Source: CAD feature listing. Evaluate the final solid. Frame: model axes, mm. Face numbers are marked on the shaded views. A direction names the side the tool comes from. Give positions to 0.01 mm unless a question says otherwise; leave off trailing zeros. Loops run counter-clockwise (first coordinate to the right, second up) from the corner with the lowest first, then second, coordinate; pieces in that order, holes last. Notation, with made-up numbers: (-21.5, 23) - (11.5, 23) arc R11 cw to (11.5, 28) - close; hole circle Ø5 at (9, 44). An arc over 180 degrees is marked (long way). Write each question's results on one line, items separated by ' | '. Start each with the question number.
(1) Cut plane A-A on x = 0. Return the cut outline in (y, z) (3 decimals).
(2) Cut plane B-B on z = -11. Return the cut outline in (x, y), then the cut area to 3 significant figures.
(3) Cut plane D-D on z = -1.5. Return the cut outline in (x, y).
(4) Contact query for flat-ended pins moving along their axis: pin 1 (1 mm diameter, centred on x = 25.5, y = -17, fed in from -Z); pin 2 (6 mm diameter, centred on x = 34.5, z = 1.5, fed in from -Y); pin 3 (4 mm diameter, centred on x = 25, y = -11, fed in from +Z). Output: stop coordinate, or through.
(5) Reachability of the marked faces 1 and 2 from +Z, -Z, +X, -X, +Y, -Y: full face, straight path, thin tool, end or side. Return the list, or none.
(6) Pull-direction query (Z, two-part tool) for the marked faces 3, 4, 5 and 6; classes: pulls with the +Z half, pulls with the -Z half, needs draft (parallel to the pull), parting line crosses it, or undercut.
(7) Material intervals for line 1 along Z through (x, y) = (0, -12) (3 decimals); line 2 along X through (y, z) = (-11, -7); line 3 along X through (y, z) = (-8.5, -1.5), sorted ascending. Write a range as [from, to].
(8) Cut plane C-C on y = -42.5. Return the cut outline in (x, z) (3 decimals), then the cut area to 3 significant figures.
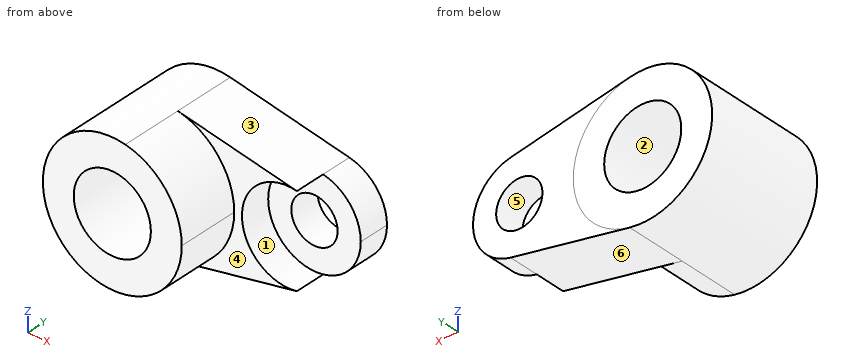
from build123d import *

# Parameters (mm, degrees)
F1_DEPTH = 25.4
F0_R     = 15.875
F2_DEPTH = 50.8
F0_R_2   = 9.525
F3_DEPTH = 12.7


with BuildPart() as f1:
    # F0 (on Front) → F1 (new body)
    with BuildSketch(Plane.XZ):
        with BuildLine():
            ThreePointArc((5.357812, 28.068211), (22.018516, 18.21306), (28.575, 0))
            ThreePointArc((28.575, 0), (22.018516, -18.21306), (5.357812, -28.068211))
            Line((5.357813, -28.068211), (54.371875, -18.712141))
            ThreePointArc((54.371875, -18.712141), (31.75, 0), (54.371875, 18.712141))
            Line((54.371875, 18.712141), (5.357812, 28.068211))
        make_face()
    extrude(amount=F1_DEPTH)

    # F0 (on Front) → F2 (join)
    with BuildSketch(Plane.XZ):
        with BuildLine():
            ThreePointArc((5.357812, -28.068211), (22.018516, -18.21306), (28.575, 0))
            ThreePointArc((28.575, 0), (22.018516, 18.21306), (5.357812, 28.068211))
            ThreePointArc((5.357812, 28.068211), (-28.575, 0), (5.357812, -28.068211))
        make_face()
        Circle(F0_R, mode=Mode.SUBTRACT)
    extrude(amount=F2_DEPTH)

    # F0 (on Front) → F3 (join)
    with BuildSketch(Plane.XZ):
        with BuildLine():
            ThreePointArc((69.85, 0), (65.479011, 12.14204), (54.371875, 18.712141))
            ThreePointArc((54.371875, 18.712141), (31.75, 0), (54.371875, -18.712141))
            ThreePointArc((54.371875, -18.712141), (65.479011, -12.14204), (69.85, 0))
        make_face()
        with Locations((50.8, 0)):
            Circle(F0_R_2, mode=Mode.SUBTRACT)
    extrude(amount=F3_DEPTH)


solid = f1.part
Ans:
1) outline: (-50.8, -28.575) - (0, -28.575) - (0, -15.875) - (-50.8, -15.875) - close; (-50.8, 15.875) - (0, 15.875) - (0, 28.575) - (-50.8, 28.575) - close
2) outline: (-26.37, -50.8) - (-11.45, -50.8) - (-11.45, 0) - (-26.37, 0) - close; (11.45, -50.8) - (26.37, -50.8) - (26.37, -25.4) - (35.25, -25.4) - (35.25, -12.7) - (66.35, -12.7) - (66.35, 0) - (11.45, 0) - close | area: 2,140 mm^2
3) outline: (-28.54, -50.8) - (-15.8, -50.8) - (-15.8, 0) - (-28.54, 0) - close; (15.8, -50.8) - (28.54, -50.8) - (28.54, -25.4) - (31.81, -25.4) - (31.81, -12.7) - (41.39, -12.7) - (41.39, 0) - (15.8, 0) - close; (60.21, -12.7) - (69.79, -12.7) - (69.79, 0) - (60.21, 0) - close
4) pin 1: z = -24.32 | pin 2: y = -25.4 | pin 3: z = 24.7
5) face 1: -Y | face 2: +Y, -Y
6) face 3: pulls with the +Z half | face 4: needs draft | face 5: undercut | face 6: pulls with the -Z half
7) line 1: [-28.575, -15.875], [15.875, 28.575] | line 2: [-27.7, -14.25], [14.25, 44.34], [57.26, 68.52] | line 3: [-28.54, -15.8], [15.8, 41.39], [60.21, 69.79]
8) outline: (5.358, -28.068) arc R28.575 ccw to (28.575, 0) arc R28.575 ccw to (5.358, 28.068) arc R28.575 ccw (long way) to start; hole circle Ø31.75 at (0, 0) | area: 1,770 mm^2
